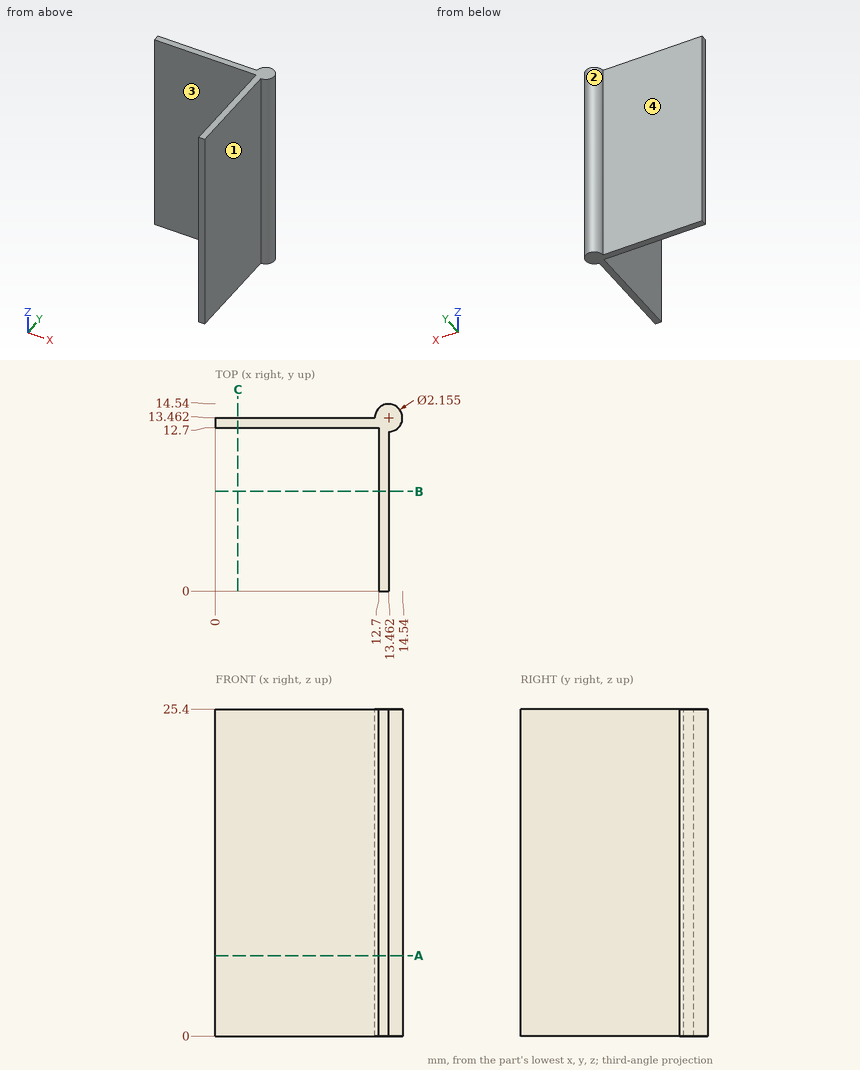
Geometry: see drawing. Coordinates: mm, zero at the bounding-box minimum. A direction names the side the tool comes from. Give positions to 0.01 mm unless a question says otherwise; leave off trailing zeros. Order: outer loops, then holes, each group sorted by start corner. A loop starts at its lowest first (then second) coordinate and runs counter-clockwise, first axis right, second up.
Q1. Section B-B on y = 7.75. Output: boundary loops of the cut face in (x, z).
Checked values:
outline: (12.7, 0) - (13.46, 0) - (13.46, 25.4) - (12.7, 25.4) - close
Q2. Contact query for flat-ended pins moving along their axis: pin 1 Ø6 at (y, z) = (4, 13.5) entering from +X; pin 2 Ø3 at (x, z) = (12, 17.5) entering from +Y; pin 3 Ø4 at (x, z) = (10, 15) entering from -Y; pin 4 Ø5 at (x, y) = (7, 8.5) entering from -Z. Output: stop coordinate, or through.
Checked values:
pin 1: stops at x = 13.46
pin 2: stops at y = 14.54
pin 3: stops at y = 12.7
pin 4: passes through
Q3. Ray query, probe 1 along Y at (x, z) = (1.25, 12.5); probe 2 along X at (y, z) = (13.75, 20). Return the intervals inside material, ascending.
Checked values:
probe 1: y = 12.7 to 13.46
probe 2: x = 12.42 to 14.5
Q4. Set-up query: the marked faces 1, 2, 3 and 4. Return all of +Z, -Z, +X, -X, +Y, -Y with unobstructed straight access to the full face (end or side cutting, diameter ignored); none if empty.
Checked values:
face 1: +Z, -Z, +X, -Y
face 2: +Z, -Z
face 3: +Z, -Z, -X, -Y
face 4: +Z, -Z, -X, +Y
Q5. Section A-A on z = 6.25. Output: boundary loops of the cut face in (x, y) (1 decimal).
Checked values:
outline: (0, 12.7) - (12.7, 12.7) - (12.7, 0) - (13.5, 0) - (13.5, 12.4) arc R1.1 ccw (long way) to (12.4, 13.5) - (0, 13.5) - close
